from build123d import *

# Parameters (mm, degrees)
F1_DEPTH = 8
F2_R     = 10


with BuildPart() as f1:
    # F0 (on Top) → F1 (new body)
    with BuildSketch(Plane.XY):
        Polygon((16.4421471655, -13.5372191966), (-45.5578528345, -13.5372191966), (-45.5578528345, -133.5372191966), (184.4421471655, -133.5372191966), (184.4421471655, -13.5372191966), (52.4421471655, -13.5372191966), (52.4421471655, -23.5372191966), (44.4421471655, -23.5372191966), (44.4421471655, -13.5372191966), (24.4421471655, -13.5372191966), (24.4421471655, -23.5372191966), (16.4421471655, -23.5372191966), align=None)
        with BuildLine():
            ThreePointArc((-30.5578528345, -114.5372191966), (-32.5578528345, -112.5372191966), (-30.5578528345, -110.5372191966))
            Line((-30.5578528345, -110.5372191966), (24.4421471655, -110.5372191966))
            ThreePointArc((24.4421471655, -110.5372191966), (26.4421471655, -112.5372191966), (24.4421471655, -114.5372191966))
            Line((24.4421471655, -114.5372191966), (-30.5578528345, -114.5372191966))
        make_face(mode=Mode.SUBTRACT)
        with BuildLine():
            ThreePointArc((-30.5578528345, -98.5372191966), (-32.5578528345, -96.5372191966), (-30.5578528345, -94.5372191966))
            Line((-30.5578528345, -94.5372191966), (24.4421471655, -94.5372191966))
            ThreePointArc((24.4421471655, -94.5372191966), (26.4421471655, -96.5372191966), (24.4421471655, -98.5372191966))
            Line((24.4421471655, -98.5372191966), (-30.5578528345, -98.5372191966))
        make_face(mode=Mode.SUBTRACT)
        with BuildLine():
            Line((24.4421471655, -82.5372191966), (-30.5578528345, -82.5372191966))
            ThreePointArc((-30.5578528345, -82.5372191966), (-32.5578528345, -80.5372191966), (-30.5578528345, -78.5372191966))
            Line((-30.5578528345, -78.5372191966), (24.4421471655, -78.5372191966))
            ThreePointArc((24.4421471655, -78.5372191966), (26.4421471655, -80.5372191966), (24.4421471655, -82.5372191966))
        make_face(mode=Mode.SUBTRACT)
        with BuildLine():
            ThreePointArc((169.4421471655, -110.5372191966), (171.4421471655, -112.5372191966), (169.4421471655, -114.5372191966))
            Line((169.4421471655, -114.5372191966), (114.4421471655, -114.5372191966))
            ThreePointArc((114.4421471655, -114.5372191966), (112.4421471655, -112.5372191966), (114.4421471655, -110.5372191966))
            Line((114.4421471655, -110.5372191966), (169.4421471655, -110.5372191966))
        make_face(mode=Mode.SUBTRACT)
        with BuildLine():
            ThreePointArc((169.4421471655, -94.5372191966), (171.4421471655, -96.5372191966), (169.4421471655, -98.5372191966))
            Line((169.4421471655, -98.5372191966), (114.4421471655, -98.5372191966))
            ThreePointArc((114.4421471655, -98.5372191966), (112.4421471655, -96.5372191966), (114.4421471655, -94.5372191966))
            Line((114.4421471655, -94.5372191966), (169.4421471655, -94.5372191966))
        make_face(mode=Mode.SUBTRACT)
        with BuildLine():
            ThreePointArc((169.4421471655, -78.5372191966), (171.4421471655, -80.5372191966), (169.4421471655, -82.5372191966))
            Line((169.4421471655, -82.5372191966), (114.4421471655, -82.5372191966))
            ThreePointArc((114.4421471655, -82.5372191966), (112.4421471655, -80.5372191966), (114.4421471655, -78.5372191966))
            Line((114.4421471655, -78.5372191966), (169.4421471655, -78.5372191966))
        make_face(mode=Mode.SUBTRACT)
        with BuildLine():
            Line((-3.0578528345, -66.5372191966), (-30.5578528345, -66.5372191966))
            ThreePointArc((-30.5578528345, -66.5372191966), (-32.5578528345, -64.5372191966), (-30.5578528345, -62.5372191966))
            Line((-30.5578528345, -62.5372191966), (-3.0578528345, -62.5372191966))
            ThreePointArc((-3.0578528345, -62.5372191966), (-1.0578528345, -64.5372191966), (-3.0578528345, -66.5372191966))
        make_face(mode=Mode.SUBTRACT)
        with BuildLine():
            Line((-3.0578528345, -50.5372191966), (-30.5578528345, -50.5372191966))
            ThreePointArc((-30.5578528345, -50.5372191966), (-32.5578528345, -48.5372191966), (-30.5578528345, -46.5372191966))
            Line((-30.5578528345, -46.5372191966), (-3.0578528345, -46.5372191966))
            ThreePointArc((-3.0578528345, -46.5372191966), (-1.0578528345, -48.5372191966), (-3.0578528345, -50.5372191966))
        make_face(mode=Mode.SUBTRACT)
        with BuildLine():
            Line((-3.0578528345, -34.5372191966), (-30.5578528345, -34.5372191966))
            ThreePointArc((-30.5578528345, -34.5372191966), (-32.5578528345, -32.5372191966), (-30.5578528345, -30.5372191966))
            Line((-30.5578528345, -30.5372191966), (-3.0578528345, -30.5372191966))
            ThreePointArc((-3.0578528345, -30.5372191966), (-1.0578528345, -32.5372191966), (-3.0578528345, -34.5372191966))
        make_face(mode=Mode.SUBTRACT)
        with BuildLine():
            ThreePointArc((169.4421471655, -62.5372191966), (171.4421471655, -64.5372191966), (169.4421471655, -66.5372191966))
            Line((169.4421471655, -66.5372191966), (141.9421471655, -66.5372191966))
            ThreePointArc((141.9421471655, -66.5372191966), (139.9421471655, -64.5372191966), (141.9421471655, -62.5372191966))
            Line((141.9421471655, -62.5372191966), (169.4421471655, -62.5372191966))
        make_face(mode=Mode.SUBTRACT)
        with BuildLine():
            ThreePointArc((169.4421471655, -46.5372191966), (171.4421471655, -48.5372191966), (169.4421471655, -50.5372191966))
            Line((169.4421471655, -50.5372191966), (141.9421471655, -50.5372191966))
            ThreePointArc((141.9421471655, -50.5372191966), (139.9421471655, -48.5372191966), (141.9421471655, -46.5372191966))
            Line((141.9421471655, -46.5372191966), (169.4421471655, -46.5372191966))
        make_face(mode=Mode.SUBTRACT)
        with BuildLine():
            ThreePointArc((169.4421471655, -30.5372191966), (171.4421471655, -32.5372191966), (169.4421471655, -34.5372191966))
            Line((169.4421471655, -34.5372191966), (141.9421471655, -34.5372191966))
            ThreePointArc((141.9421471655, -34.5372191966), (139.9421471655, -32.5372191966), (141.9421471655, -30.5372191966))
            Line((141.9421471655, -30.5372191966), (169.4421471655, -30.5372191966))
        make_face(mode=Mode.SUBTRACT)
    extrude(amount=F1_DEPTH)

    # F2
    f2_edges = [f1.edges().sort_by_distance(p)[0] for p in [
        (-45.557853, -133.537219, 4),
        (184.442147, -133.537219, 4),
    ]]
    fillet(f2_edges, radius=F2_R)


solid = f1.part
Could you check a few things on this model? Use its own coordinates, in mm. A direction names the side the tool comes from. Coordinates: 2 decimals unless noted, no trailing zeros. Order: outer loops, then holes, each group sorted by start corner. A loop starts at its lowest first (then second) coordinate and runs counter-clockwise, first axis right, second up.
Q1. Suppose I cut it at B-B on x = 146. Please give me the cut outline in (y, z).
Q2. Please list where these lines run through material, in increasing order: L1, parallel to Y at x = 131.5, z = 4.5; L2, parallel to X at y = -79, z = 5.25; L3, parallel to X at y = -66, z = 4.75.
Q3. Will this pin go through, and if not, where does the flat tip stop? pin 1 (2.5 mm diameter, centred on x = 47.5, z = 3, fed in from +Y).
Q4. Thinking about a two-plate mould opening in Y: for faces 1 (the flat face through (68, -73, 0)), 2 (the cylindrical face through (171.44, -32.49, 3.94)), 3 (the flat face through (-3, -82.537, 4)), which applies, released by +Y, released by -Y, zero draft, split by the parting line, or undercut?
Q5. Suppose I cut it at A-A on x = 13.5. Please give me the cut outline in (y, z).
Q6. Suppose I cut it at C-C on z = 6.75. Give the number of separate pieces and of enclosed holes in the cut face, and give its area (3 significant figures).
Q7. Which directions (+Z, -Z, +X, -X, +Y, -Y) give clear straight access to the entire face, cutting with the end or side of a thin tool? Please do faces 4 (the cylindrical face through (26.44, -96.49, 3.94)), 5 (the flat face through (52.442, -18, 4)).
Answer:
1. outline: (-133.54, 0) - (-114.54, 0) - (-114.54, 8) - (-133.54, 8) - close; (-110.54, 0) - (-98.54, 0) - (-98.54, 8) - (-110.54, 8) - close; (-94.54, 0) - (-82.54, 0) - (-82.54, 8) - (-94.54, 8) - close; (-78.54, 0) - (-66.54, 0) - (-66.54, 8) - (-78.54, 8) - close; (-62.54, 0) - (-50.54, 0) - (-50.54, 8) - (-62.54, 8) - close; (-46.54, 0) - (-34.54, 0) - (-34.54, 8) - (-46.54, 8) - close; (-30.54, 0) - (-13.54, 0) - (-13.54, 8) - (-30.54, 8) - close
2. L1: y = -133.54 to -114.54, -110.54 to -98.54, -94.54 to -82.54, -78.54 to -13.54
2. L2: x = -45.56 to -31.84, 25.72 to 113.16, 170.72 to 184.44
2. L3: x = -45.56 to -31.92, -1.69 to 140.58, 170.81 to 184.44
3. pin 1: stops at y = -23.54
4. face 1: zero draft
4. face 2: undercut
4. face 3: undercut
5. outline: (-133.54, 0) - (-114.54, 0) - (-114.54, 8) - (-133.54, 8) - close; (-110.54, 0) - (-98.54, 0) - (-98.54, 8) - (-110.54, 8) - close; (-94.54, 0) - (-82.54, 0) - (-82.54, 8) - (-94.54, 8) - close; (-78.54, 0) - (-13.54, 0) - (-13.54, 8) - (-78.54, 8) - close
6. separate pieces: 1
6. enclosed holes: 12
6. area: 25,300 mm2
7. face 4: +Z, -Z
7. face 5: +Z, -Z, +Y
